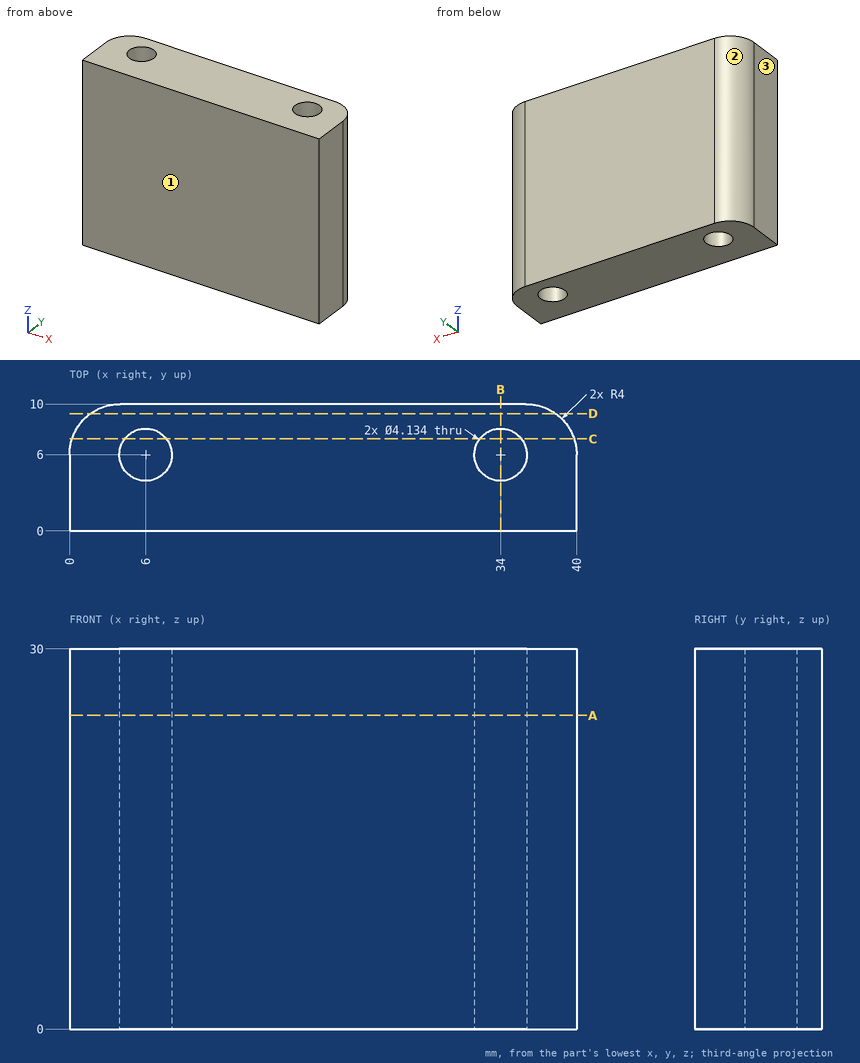
For this review, use the dimensioned drawing (mm, ordinates from the lowest corner) and the shaded views. Coordinates: 2 decimals unless noted, no trailing zeros. Loops run counter-clockwise (first coordinate to the right, second up) from the corner with the lowest first, then second, coordinate; pieces in that order, holes last. Notation, with made-up numbers: (39, 39) - (70, 39) arc R12 cw to (70, 61) - close; hole circle Ø5 at (13.5, 54). An arc over 180 degrees is marked (long way). Use one line per item in the form item = value. Start each with the question number.
1) For pin 1 (5.5 mm diameter, centred on x = 34, y = 6, fed in from -Z), flat-tipped, find the tip position at first contact; note if it passes through.
2) Take a section at C-C (y = 7.25). State the section outline as (x, z) points.
3) To check wall thickness, follow probe 1 along X at (y, z) = (6, 19.75); probe 2 along Y at (x, z) = (6, 13.5); probe 3 along Y at (x, z) = (32.5, 3.25). State the ranges of each line that lie inside material, in increasing order. Write a range as from..to.
4) Draft analysis for pull direction Y (two halves, no side actions). For the marked faces 1, 2 and 3, state which applies: released by +Y, released by -Y, zero draft, split by the parting line, or undercut.
5) Take a section at A-A (z = 24.75). State the section outline as (x, y) points.
6) Take a section at B-B (x = 34). State the section outline as (y, z) points, plus the area to 3 significant figures.
7) Take a section at D-D (y = 9.25). State the section outline as (x, z) points.
From the geometry:
q1.pin_1 = 0
q2.outline = (0.2, 0) - (4.35, 0) - (4.35, 30) - (0.2, 30) - close; (7.65, 0) - (32.35, 0) - (32.35, 30) - (7.65, 30) - close; (35.65, 0) - (39.8, 0) - (39.8, 30) - (35.65, 30) - close
q3.probe_1 = 0..3.93, 8.07..31.93, 36.07..40
q3.probe_2 = 0..3.93, 8.07..10
q3.probe_3 = 0..4.58, 7.42..10
q4.face_1 = released by -Y
q4.face_2 = released by +Y
q4.face_3 = zero draft
q5.outline = (0, 0) - (40, 0) - (40, 6) arc R4 ccw to (36, 10) - (4, 10) arc R4 ccw to (0, 6) - close; hole circle Ø4.13 at (6, 6); hole circle Ø4.13 at (34, 6)
q6.outline = (0, 0) - (3.93, 0) - (3.93, 30) - (0, 30) - close; (8.07, 0) - (10, 0) - (10, 30) - (8.07, 30) - close
q6.area = 176 mm2
q7.outline = (1.67, 0) - (38.33, 0) - (38.33, 30) - (1.67, 30) - close
